```python
from build123d import *

# Parameters (mm, degrees)
SKETCH2_W               = 40.64
SKETCH2_H               = 127
BOSS_EXTRUDE1_DEPTH     = 6.35
M6_CLEARANCE_HOLE1_D    = 6.6
CUT_EXTRUDE1_DEPTH      = 134.495063954
CUT_EXTRUDE1_DEPTH_BACK = 134.495063954
SKETCH5_W               = 7.0505
SKETCH5_H               = 127
SKETCH6_W               = 27.8745
SKETCH6_H               = 3.175
CUT_EXTRUDE2_DEPTH      = 134.495063954
SKETCH7_W               = 6.35
SKETCH7_H               = 4.7625
CUT_EXTRUDE3_DEPTH      = 134.495063954


with BuildPart() as part:
    # Sketch2 → Boss-Extrude1 (new body)
    with BuildSketch(Plane.XY):
        with Locations((20.32, 63.5)):
            Rectangle(SKETCH2_W, SKETCH2_H)
    extrude(amount=BOSS_EXTRUDE1_DEPTH)

    # M6 Clearance Hole1 (through all)
    with Locations(Plane.XY.offset(6.35)):
        with Locations((17.4625, 31.75), (17.4625, 95.25)):
            Hole(M6_CLEARANCE_HOLE1_D / 2)

    # Sketch5 → Cut-Extrude1 (cut, two sides: drawn at the far end of the back side and taken through both)
    with BuildSketch(Plane.XY.offset(6.35).offset(-CUT_EXTRUDE1_DEPTH_BACK)):
        with Locations((3.52525, 63.5)):
            Rectangle(SKETCH5_W, SKETCH5_H)
    extrude(amount=CUT_EXTRUDE1_DEPTH + CUT_EXTRUDE1_DEPTH_BACK, mode=Mode.SUBTRACT)

    # Sketch6 → Cut-Extrude2 (cut, through all)
    with BuildSketch(Plane.XY.offset(6.35)):
        Polygon((7.0505, 123.825), (7.0505, 120.65), (37.30625, 120.65), (37.30625, 127), (34.925, 127), (34.925, 123.825), align=None)
        with Locations((20.98775, 125.4125)):
            Rectangle(SKETCH6_W, SKETCH6_H)
        Polygon((37.30625, 66.675), (7.0505, 66.675), (7.0505, 63.5), (34.925, 63.5), (34.925, 60.325), (7.0505, 60.325), (7.0505, 57.15), (37.30625, 57.15), align=None)
        with Locations((20.98775, 61.9125)):
            Rectangle(SKETCH6_W, SKETCH6_H)
        Polygon((37.30625, 0), (37.30625, 6.35), (7.0505, 6.35), (7.0505, 3.175), (34.925, 3.175), (34.925, 0), align=None)
        with Locations((20.98775, 1.5875)):
            Rectangle(SKETCH6_W, SKETCH6_H)
    extrude(amount=-CUT_EXTRUDE2_DEPTH, mode=Mode.SUBTRACT)

    # Sketch7 → Cut-Extrude3 (cut, through all)
    with BuildSketch(Plane.XY.offset(6.35)):
        with Locations((31.115, 118.26875)):
            Rectangle(SKETCH7_W, SKETCH7_H)
        with Locations((31.115, 69.05625)):
            Rectangle(SKETCH7_W, SKETCH7_H)
        with Locations((31.115, 54.76875)):
            Rectangle(SKETCH7_W, SKETCH7_H)
        with Locations((31.115, 8.73125)):
            Rectangle(SKETCH7_W, SKETCH7_H)
    extrude(amount=-CUT_EXTRUDE3_DEPTH, mode=Mode.SUBTRACT)


solid = part.part
```
Part model, mm, in its own coordinate system. A direction names the side the tool comes from. Round coordinates to 2 decimals unless told otherwise and drop trailing zeros. Loops run counter-clockwise (first coordinate to the right, second up) from the corner with the lowest first, then second, coordinate; pieces in that order, holes last.
Item 1: Drop flat-ended pins along their axis: P1, Ø8, axis at x = 16, y = 50.5, coming from the -Z side; P2, Ø3, axis at x = 31, z = 4.5, coming from the -Y side; P3, Ø1.9, axis at x = 19.5, z = 3.5, coming from the +Y side; P4, Ø3, axis at y = 122.5, z = 3.5, coming from the -X side. Give the stop position or say it passes through.
Item 2: Cut at A-A, the plane x = 33. Give the cut face in (y, z).
Item 3: Drill centre lines: line 1 (Y direction, x = 26, z = 5) (3 decimals); line 2 (Y direction, x = 20, z = 4.25) (3 decimals); line 3 (X direction, y = 8, z = 3.5). Where is each one in solid material? Low to high.
Item 4: Cut at C-C, the plane z = 1. State how many separate pieces and enclosed holes the cut face has, then the cut area to 3 significant figures.
Item 5: Cut at D-D, the plane x = 15.5. Give the cut face in (y, z) (3 decimals).
Item 6: 3-axis set-ups, long thin cutter, end or side, ignore diameter. For faces 5 (the face through (36, 66.675, 3)), 6 (the face through (34.29, 9, 3)), 7 (the face through (17, 120.65, 3)): which of +Z, -Z, +X, -X, +Y, -Y reach the whole face in a straight line?
Item 7: Cut at B-B, the plane y = 31.75. Give the cut face in (x, z).
Item 8: Mould opens along X. For faces 1 (the face through (18, 6.35, 3)), 2 (the face through (31, 11.112, 3)), 3 (the face through (40.64, 63, 3)), 4 (the face through (27.94, 69, 3)) say: +X half, -X half, draft (parallel to the pull), parting line (faces both ways), or undercut.
A:
1. P1: stops at z = 0
1. P2: stops at y = 11.11
1. P3: stops at y = 120.65
1. P4: stops at x = 37.31
2. outline: (11.11, 0) - (52.39, 0) - (52.39, 6.35) - (11.11, 6.35) - close; (71.44, 0) - (115.89, 0) - (115.89, 6.35) - (71.44, 6.35) - close
3. line 1: y = 6.35 to 57.15, 66.675 to 120.65
3. line 2: y = 6.35 to 29.64, 33.86 to 57.15, 66.675 to 93.14, 97.36 to 120.65
3. line 3: x = 7.05 to 27.94, 34.29 to 40.64
4. separate pieces: 1
4. enclosed holes: 2
4. area: 3,400 mm2
5. outline: (6.35, 0) - (29.097, 0) - (29.097, 6.35) - (6.35, 6.35) - close; (34.403, 0) - (57.15, 0) - (57.15, 6.35) - (34.403, 6.35) - close; (66.675, 0) - (92.597, 0) - (92.597, 6.35) - (66.675, 6.35) - close; (97.903, 0) - (120.65, 0) - (120.65, 6.35) - (97.903, 6.35) - close
6. face 5: +Z, -Z, -X
6. face 6: +Z, -Z, -Y
6. face 7: +Z, -Z, -X, +Y
7. outline: (7.05, 0) - (14.16, 0) - (14.16, 6.35) - (7.05, 6.35) - close; (20.76, 0) - (40.64, 0) - (40.64, 6.35) - (20.76, 6.35) - close
8. face 1: draft
8. face 2: undercut
8. face 3: +X half
8. face 4: undercut
